```python
from build123d import *

# Parameters (mm, degrees)
SKETCH1_W                 = 32.5
SKETCH1_H                 = 42
BOSS_EXTRUDE2_DEPTH       = 3
F_2_56_TAPPED_HOLE1_D     = 1.778
F_2_56_TAPPED_HOLE1_DEPTH = 5.19583491
F_2_56_TAPPED_HOLE1_TIP   = 0.53416509
F_2_56_TAPPED_HOLE2_D     = 1.778
F_2_56_TAPPED_HOLE2_DEPTH = 5.19583491
F_2_56_TAPPED_HOLE2_TIP   = 0.53416509
CUT_EXTRUDE1_DEPTH        = 3
SKETCH10_W                = 10
SKETCH10_H                = 6.5
CUT_EXTRUDE2_DEPTH        = 1.5


with BuildPart() as part:
    # Sketch1 → Boss-Extrude2 (new body)
    with BuildSketch(Plane.XY):
        with Locations((16.25, 21)):
            Rectangle(SKETCH1_W, SKETCH1_H)
    extrude(amount=BOSS_EXTRUDE2_DEPTH)

    # #2-56 Tapped Hole1
    with Locations(Plane.ZY):
        with Locations((1.5, 33), (1.5, 9)):
            Hole(F_2_56_TAPPED_HOLE1_D / 2, depth=F_2_56_TAPPED_HOLE1_DEPTH)
            with Locations((0, 0, -(F_2_56_TAPPED_HOLE1_DEPTH + F_2_56_TAPPED_HOLE1_TIP / 2))):  # 118° drill point
                Cone(0, F_2_56_TAPPED_HOLE1_D / 2, F_2_56_TAPPED_HOLE1_TIP, mode=Mode.SUBTRACT)

    # #2-56 Tapped Hole2
    with Locations(Plane(origin=(32.5, 0, 0), x_dir=(0, 0, -1), z_dir=(1, 0, 0))):
        with Locations((-1.5, 33), (-1.5, 9)):
            Hole(F_2_56_TAPPED_HOLE2_D / 2, depth=F_2_56_TAPPED_HOLE2_DEPTH)
            with Locations((0, 0, -(F_2_56_TAPPED_HOLE2_DEPTH + F_2_56_TAPPED_HOLE2_TIP / 2))):  # 118° drill point
                Cone(0, F_2_56_TAPPED_HOLE2_D / 2, F_2_56_TAPPED_HOLE2_TIP, mode=Mode.SUBTRACT)

    # Sketch9 → Cut-Extrude1 (cut)
    with BuildSketch(Plane(origin=(0, 0, 0), x_dir=(-1, 0, 0), z_dir=(0, 0, -1))):
        with BuildLine():
            ThreePointArc((-11.4, 21), (-8.4, 18), (-5.4, 21))
            Line((-5.4, 21), (-8.4, 21))
            Line((-8.4, 21), (-11.4, 21))
        make_face()
        with BuildLine():
            Line((-8.4, 21), (-5.4, 21))
            ThreePointArc((-5.4, 21), (-8.4, 24), (-11.4, 21))
            Line((-11.4, 21), (-8.4, 21))
        make_face()
    extrude(amount=-CUT_EXTRUDE1_DEPTH, mode=Mode.SUBTRACT)

    # Sketch10 → Cut-Extrude2 (cut)
    with BuildSketch(Plane(origin=(0, 0, 0), x_dir=(-1, 0, 0), z_dir=(0, 0, -1))):
        with Locations((-16.25, 38.75)):
            Rectangle(SKETCH10_W, SKETCH10_H)
    extrude(amount=-CUT_EXTRUDE2_DEPTH, mode=Mode.SUBTRACT)


solid = part.part
```
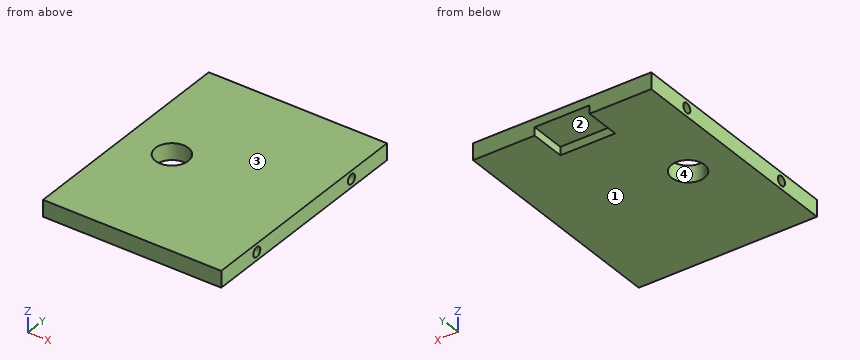
Input: part model. Units: mm. Frame: model coordinates. Face numbers are marked on the shaded views. A direction names the side the tool comes from. Coordinates: 2 decimals unless noted, no trailing zeros. Write each loop counter-clockwise with the first axis right and the second up, starting at its lowest first coordinate (ties: lowest second). Pieces come first, ordered by that corner, then holes. Notation, with made-up numbers: (46.25, 61) -> (60.25, 61) arc R15 ccw to (60.25, 83) -> close; hole circle Ø11 at (-10.5, 43). An arc over 180 degrees is marked (long way). Write each question's results on one line, items separated by ' | '.
Item 1: Section query A-A on y = 21. Return loops of the section in (x, z), plus the area to 3 significant figures.
Conclusion:
outline: (0, 0) -> (5.4, 0) -> (5.4, 3) -> (0, 3) -> close; (11.4, 0) -> (32.5, 0) -> (32.5, 3) -> (11.4, 3) -> close | area: 79.5 mm^2
Item 2: Pin query (flat end, axial travel): pin 1 Ø1.6 at (x, z) = (16, 0.5) entering from +Y; pin 2 Ø1.1 at (y, z) = (9, 1.5) entering from +X; pin 3 Ø1.4 at (y, z) = (33, 1.5) entering from -X. Return the tip coordinate at first contact, or that it passes through.
Conclusion:
pin 1: stops at y = 35.5 | pin 2: stops at x = 27.1 | pin 3: stops at x = 5.31
Item 3: Section query C-C on y = 38. Return loops of the section in (x, z).
Conclusion:
outline: (0, 0) -> (11.25, 0) -> (11.25, 1.5) -> (21.25, 1.5) -> (21.25, 0) -> (32.5, 0) -> (32.5, 3) -> (0, 3) -> close
Item 4: Section query B-B on x = 8.4. Return loops of the section in (y, z), plus the area to 3 significant figures.
Conclusion:
outline: (0, 0) -> (18, 0) -> (18, 3) -> (0, 3) -> close; (24, 0) -> (42, 0) -> (42, 3) -> (24, 3) -> close | area: 108 mm^2
Item 5: Mould query, pull axis Y, two halves, no side actions, for the marked faces 3 and 4. Classes: +Y half, -Y half, draft (parallel to the pull), parting line (faces both ways), or undercut.
Conclusion:
face 3: draft | face 4: undercut
Item 6: Material intervals for probe 1 along Y at (x, z) = (1.05, 1.5); probe 2 along Z at (x, y) = (2.65, 9); probe 3 along X at (y, z) = (38, 1), sorted ascending.
Conclusion:
probe 1: y = 0 to 8.11, 9.89 to 32.11, 33.89 to 42 | probe 2: z = 0 to 0.61, 2.39 to 3 | probe 3: x = 0 to 11.25, 21.25 to 32.5
Item 7: Set-up query: the marked faces 1 and 2. Return all of +Z, -Z, +X, -X, +Y, -Y with unobstructed straight access to the full face (end or side cutting, diameter ignored); none if empty.
Conclusion:
face 1: -Z, +X, -X, +Y, -Y | face 2: -Z, +Y
Item 8: Section query D-D on x = 16. Return loops of the section in (y, z).
Conclusion:
outline: (0, 0) -> (35.5, 0) -> (35.5, 1.5) -> (42, 1.5) -> (42, 3) -> (0, 3) -> close
